from build123d import *

# Parameters (mm, degrees)
SKETCH_1_R                       = 27.5
EXTRUDE_1_DEPTH                  = 17
SKETCH_2_R                       = 13
EXTRUDE_2_DEPTH                  = 4
EXTRUDE_START                    = 4
SKETCH_3_R                       = 13
EXTRUDE_3_DEPTH                  = 4
HOLE_WIZARD_M5_1_D               = 4.2
CUT_EXTRUDE_4_DEPTH              = 45.198416261
FILLET_1_R                       = 6
PATTERN_CIRCULAR_1_COUNT         = 2
PATTERN_CIRCULAR_1_ANGLE         = 120
FILLET_1_OF_PATTERN_CIRCULAR_1_R = 6
PATTERN_CIRCULAR_2_DEPTH         = 17
PATTERN_CIRCULAR_3_COUNT         = 3
SKETCH_15_R                      = 12
EXTRUDE_4_DEPTH                  = 9
SKETCH_16_R                      = 6
CUT_EXTRUDE_5_DEPTH              = 34
SKETCH_17_W                      = 4
SKETCH_17_H                      = 2.143145751
CUT_EXTRUDE_6_DEPTH              = 34


# Read off the part's stored shape, not the designer's step: 阵列(圆周)2
with BuildPart() as part:
    # 草图1 → 凸台-拉伸1 (new body)
    with BuildSketch(Plane.XY):
        Circle(SKETCH_1_R)
    extrude(amount=EXTRUDE_1_DEPTH)

    # 草图2 → 凸台-拉伸2 (add)
    with BuildSketch(Plane(origin=(0, 0, 0), x_dir=(-1, 0, 0), z_dir=(0, 0, -1))):
        with Locations(Location((0, 0, 0), (0, 0, 180))):
            Circle(SKETCH_2_R)
    extrude(amount=EXTRUDE_2_DEPTH)

    # 草图3 → 凸台-拉伸3 (add)
    with BuildSketch(Plane.XY.offset(17).offset(EXTRUDE_START)):
        Circle(SKETCH_3_R)
    extrude(amount=-EXTRUDE_3_DEPTH)

    # M5 螺纹孔1 (through all)
    with Locations(Plane(origin=(16.263455967, -16.263455967, 17), x_dir=(1, 0, 0), z_dir=(0, 0, 1))):
        with Locations((0, 0), (5.952838038, 10.31061793)):
            hole_wizard_m5_1 = Hole(HOLE_WIZARD_M5_1_D / 2)

    # 草图14 → 切除-拉伸4 (cut, through all)
    with BuildSketch(Plane.XY.offset(17)):
        Polygon((0, -23), (0, -20), (-15.074813432, -23), align=None)
        Polygon((15.074813432, -23), (0, -20), (0, -23), align=None)
        with BuildLine():
            Line((15.074813432, -23), (0, -23))
            Line((0, -23), (-15.074813432, -23))
            ThreePointArc((-15.074813432, -23), (0, -27.5), (15.074813432, -23))
        make_face()
    cut_extrude_4 = extrude(amount=-CUT_EXTRUDE_4_DEPTH, mode=Mode.SUBTRACT)

    # 圆角1
    fillet_1_edges = [part.edges().sort_by_distance(p)[0] for p in [
        (15.074813432, -23, 8.5),
        (-15.074813432, -23, 8.5),
        (0, -20, 8.5),
    ]]
    fillet(fillet_1_edges, radius=FILLET_1_R)

    # 阵列(圆周)1: 切除-拉伸4 ×2 about axis
    pattern_circular_1_axis = Axis((0, 0, 0), (0, 0, 1))
    for i in range(1, PATTERN_CIRCULAR_1_COUNT):
        add(cut_extrude_4.rotate(pattern_circular_1_axis, i * PATTERN_CIRCULAR_1_ANGLE / (PATTERN_CIRCULAR_1_COUNT - 1)), mode=Mode.SUBTRACT)

    # 圆角1 of 阵列(圆周)1
    fillet_1_of_pattern_circular_1_edges = [part.edges().sort_by_distance(p)[0] for p in [
        (12.381177571, 24.555171389, 8.5),
        (27.455991003, -1.555171389, 8.5),
        (17.320508076, 10, 8.5),
    ]]
    fillet(fillet_1_of_pattern_circular_1_edges, radius=FILLET_1_OF_PATTERN_CIRCULAR_1_R)

    # 阵列(圆周)2 outline → 阵列(圆周)2 (cut)
    with BuildSketch(Plane.XY):
        with BuildLine():
            Line((-16.936798412, 11.13071193), (-13.227796767, 22.060362126))
            ThreePointArc((-13.227796767, 22.060362126), (-11.854885653, 24.30763066), (-9.651911166, 25.750545836))
            ThreePointArc((-9.651911166, 25.750545836), (-23.815698604, 13.75), (-27.126582438, -4.516472653))
            ThreePointArc((-27.126582438, -4.516472653), (-26.978468484, -1.887183196), (-25.718732401, 0.425426973))
            Line((-25.718732401, 0.425426973), (-18.107878499, 9.102341718))
            ThreePointArc((-18.107878499, 9.102341718), (-17.422403117, 10.05882913), (-16.936798412, 11.13071193))
        make_face()
    extrude(amount=PATTERN_CIRCULAR_2_DEPTH, mode=Mode.SUBTRACT)

    # 阵列(圆周)3: M5 螺纹孔1 ×3 about axis
    pattern_circular_3_axis = Axis((0, 0, 0), (0, 0, 1))
    for i in range(1, PATTERN_CIRCULAR_3_COUNT):
        add(hole_wizard_m5_1.rotate(pattern_circular_3_axis, i * 360 / PATTERN_CIRCULAR_3_COUNT), mode=Mode.SUBTRACT)

    # 草图15 → 凸台-拉伸4 (add)
    with BuildSketch(Plane.XY.offset(21)):
        Circle(SKETCH_15_R)
    extrude(amount=EXTRUDE_4_DEPTH)

    # 草图16 → 切除-拉伸5 (cut)
    with BuildSketch(Plane.XY.offset(30)):
        Circle(SKETCH_16_R)
    extrude(amount=-CUT_EXTRUDE_5_DEPTH, mode=Mode.SUBTRACT)

    # 草图17 → 切除-拉伸6 (cut)
    with BuildSketch(Plane.XY.offset(30)):
        with Locations((0, 6.728427125)):
            Rectangle(SKETCH_17_W, SKETCH_17_H)
    extrude(amount=-CUT_EXTRUDE_6_DEPTH, mode=Mode.SUBTRACT)


solid = part.part
Design review of the part built by this model. Coordinates are the model's own, in mm. A direction names the side the tool comes from. Coordinates: 2 decimals unless noted, no trailing zeros. Write each loop counter-clockwise with the first axis right and the second up, starting at its lowest first coordinate (ties: lowest second). Pieces come first, ordered by that corner, then holes. Notation, with made-up numbers: (69.5, -25.75) - (118.5, -25.75) arc R13 ccw to (118.5, -11.75) - close; hole circle Ø4 at (-17, -34). An arc over 180 degrees is marked (long way). One line per item, written item: value.
1) Mouldability with a two-part tool opening along Y and no side actions: class faces 6 (the face through (26.989, -1.923, 8.381)), 7 (the face through (4.824, 23.987, 8.381)), 8 (the face through (-15.2, -22.4, 8.4)), 9 (the face through (-15.99, -14.18, 8.38)) as +Y half, -Y half, draft (parallel to the pull), parting line (faces both ways), or undercut.
Answer sheet:
face 6: parting line
face 7: undercut
face 8: -Y half
face 9: undercut
2) To check wall thickness, follow probe 1 along Y at (x, z) = (0, 14.5); probe 2 along Z at (x, y) = (-17, 1); probe 3 along Y at (x, z) = (18, 6). State the ranges of each line that lie inside material, in increasing order.
Answer sheet:
probe 1: y = -20.12 to -6, 7.8 to 27.5
probe 2: z = 0 to 17
probe 3: y = -20.79 to -17.44, -15.08 to 9.23
3) Insertion check: pin 1 (2.5 mm diameter, centred on x = -22.22, y = -5.95, fed in from +Z); pin 2 (6.5 mm diameter, centred on x = 5.95, y = 22.22, fed in from +Z); pin 3 (4.5 mm diameter, centred on x = -0.5, z = 6, fed in from -Y); pin 4 (2.5 mm diameter, centred on y = 7.5, z = 14, fed in from -X). Each pin has a flat end and moves straight along its axis. Give the tip position at first contact, or say it passes through.
Answer sheet:
pin 1: passes through
pin 2: stops at z = 17
pin 3: stops at y = -20.55
pin 4: stops at x = -20.61
4) Add section C-C (y = 10). State the section outline as (x, z) points.
Answer sheet:
outline: (-17.46, 0) - (-8.31, 0) - (-8.31, -4) - (8.31, -4) - (8.31, 0) - (17.46, 0) - (17.46, 17) - (8.31, 17) - (8.31, 21) - (6.63, 21) - (6.63, 30) - (-6.63, 30) - (-6.63, 21) - (-8.31, 21) - (-8.31, 17) - (-17.46, 17) - close
5) For faces 1 (the face through (2, 7, 13)), 2 (the face through (0, -14, 0)), 3 (the face through (21.86, 4.825, 8.619)), 4 (the face through (-6.752, -21.344, 8.619)), 5 (the face through (-11.99, 0.53, 25.44)), list the 3-axis set-ups (+Z, -Z, +X, -X, +Y, -Y) from which the entire face can be reached by the end or side of a thin tool; tool diameter is ignored.
Answer sheet:
face 1: +Z, -Z
face 2: -Z
face 3: +Z, -Z, +X, +Y
face 4: +Z, -Z, -Y
face 5: +Z
6) Add section B-B (z = 25). State the section outline as (x, y) points, plus the area to 3 significant figures.
Answer sheet:
outline: circle Ø24 at (0, 0); hole (-2, 5.66) arc R6 ccw (long way) to (2, 5.66) - (2, 7.8) - (-2, 7.8) - close
area: 332 mm2
7) Add section A-A (x = 0). State the section outline as (y, z) points.
Answer sheet:
outline: (-20.12, 0) - (-13, 0) - (-13, -4) - (-6, -4) - (-6, 30) - (-12, 30) - (-12, 21) - (-13, 21) - (-13, 17) - (-20.12, 17) - close; (7.8, -4) - (13, -4) - (13, 0) - (27.5, 0) - (27.5, 17) - (13, 17) - (13, 21) - (12, 21) - (12, 30) - (7.8, 30) - close
8) Add section D-D (z = 20). State the section outline as (x, y) points.
Answer sheet:
outline: circle Ø26 at (0, 0); hole (-2, 5.66) arc R6 ccw (long way) to (2, 5.66) - (2, 7.8) - (-2, 7.8) - close
